Study the drawing (mm; zero at the part's minimum x, y, z) and answer. Coordinates: 2 decimals unless noted, no trailing zeros. Write each loop counter-clockwise with the first axis right and the second up, starting at its lowest first coordinate (ties: lowest second). Pieces come first, ordered by that corner, then holes. Notation, with made-up numbers: (-26.75, 16) -> (26.25, 16) arc R26 ccw to (26.25, 48) -> close; hole circle Ø2 at (25, 79). An arc over 180 degrees is marked (long way). Answer in a Markdown table with one row per item. Add a question column.
Item 1: Section A-A on y = 6 is taken. Write down the section's boundary in (x, z).
Item 2: Section C-C on x = 20.5 is taken. Write down the section's boundary in (y, z), then the cut area to 3 significant figures.
Item 3: Straight lines are drawn through the part: line 1 (Y direction, x = 37, z = 31); line 2 (Z direction, x = 32.5, y = 7); line 3 (X direction, y = 5, z = 35). For each, find the intervals that lie inside material, in ascending order. Write a range as from..to.
Item 4: Given pin 1 Ø10 at (y, z) = (33, 47.5) entering from -X; pin 2 Ø12.5 at (x, z) = (29, 38.5) entering from -Y, each flat-ended and moving along its own axis, determine where each tip first touches the part or whether it passes through.
Item 5: Section B-B on z = 38 is taken. Write down the section's boundary in (x, y) (1 decimal), then the cut area to 3 significant figures.
Item 6: For a pull along Z with two mould halves and no side action, classify the marked faces 1, 2 and 3 as +Z half, -Z half, draft (parallel to the pull), parting line (faces both ways), or undercut.
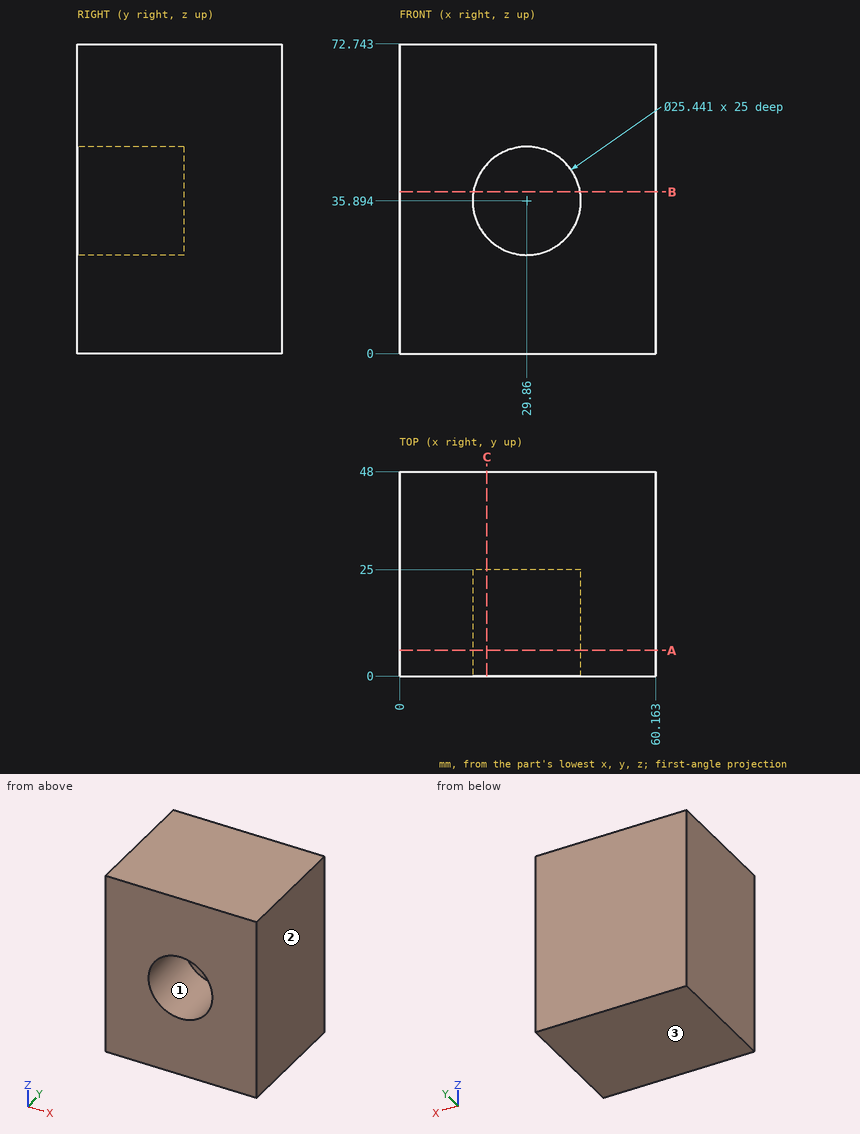
Results below:
| question | item | result |
|---|---|---|
| 1 | outline | (0, 0) -> (60.16, 0) -> (60.16, 72.74) -> (0, 72.74) -> close; hole circle Ø25.44 at (29.86, 35.89) |
| 2 | outline | (0, 0) -> (48, 0) -> (48, 72.74) -> (0, 72.74) -> (0, 44.51) -> (25, 44.51) -> (25, 27.28) -> (0, 27.28) -> close |
| 2 | area | 3,060 mm2 |
| 3 | line 1 | y = 25..48 |
| 3 | line 2 | z = 0..23.45, 48.34..72.74 |
| 3 | line 3 | x = 0..17.17, 42.55..60.16 |
| 4 | pin 1 | stops at x = 0 |
| 4 | pin 2 | stops at y = 25 |
| 5 | outline | (0, 0) -> (17.3, 0) -> (17.3, 25) -> (42.4, 25) -> (42.4, 0) -> (60.2, 0) -> (60.2, 48) -> (0, 48) -> close |
| 5 | area | 2,260 mm2 |
| 6 | face 1 | undercut |
| 6 | face 2 | draft |
| 6 | face 3 | -Z half |
